The listing builds one solid part. Answer for the finished solid, in the listing's coordinates (mm). A direction names the side the tool comes from. Round coordinates to 2 decimals unless told otherwise and drop trailing zeros. Write each loop counter-clockwise with the first axis right and the second up, starting at its lowest first coordinate (ties: lowest second). Pieces come first, ordered by that corner, then holes. Notation, with made-up numbers: (-12, -24) - (36, -24) arc R20 ccw to (36, -5) - close; hole circle Ø2 at (46, -18). An arc over 180 degrees is marked (long way). Use a Markdown table: item, result. Add a question column.
1) A cutting plane is placed at D-D (y = -11.5). Give the vertices of the cut face in (x, z) (3 decimals).
2) Each of these flat-tipped pins is pushed along its axis until it touches: P1, Ø3, axis at x = 8, z = 4.62, coming from the -Y side; P2, Ø10, axis at y = 10.5, z = -8, coming from the -X side; P3, Ø6, axis at x = 8, z = -2, coming from the +Y side; P4, Ø6, axis at x = -5, y = 13.5, coming from the +Z side. Where does it stop, or does it pass through?
3) Determine the mould class of faces 1 (the flat face through (5, -11.04, 5)), 2 (the cylindrical face through (-0.1, 15.1, 2.5)), 3 (the flat face through (0, 17.56, 3)) for opening direction Y: +Y half, -Y half, draft (parallel to the pull), parting line (faces both ways), or undercut.
4) A tool of negligible diameter and unlimited length cuts with its end or side. For faces 4 (the flat face through (0, -17.56, -3)), 5 (the cylindrical face through (-1.951, 16.292, -6.195)), 6 (the cylindrical face through (3.955, -0.155, 5.158)), from which of +Z, -Z, +X, -X, +Y, -Y can it reach the whole face along a straight path? Write none if from no direction.
5) Find the intervals of material crossed by probe 1 along Y at (x, z) = (-4.75, -7.75); probe 2 along Z at (x, y) = (0.25, 4.5); probe 3 along X at (y, z) = (-12, 0.25), in increasing order. Write a range as from..to.
6) A cutting plane is placed at C-C (x = -8). Give the vertices of the cut face in (y, z).
```python
from build123d import *

# Parameters (mm, degrees)
FORO_FILETTATO_M3X0_5_1_D = 2.5


with BuildPart() as part:
    # Schizzo1 → Rivoluzione1 (revolve)
    with BuildSketch(Plane.XY, mode=Mode.PRIVATE) as rivoluzione1_sk:
        Polygon((2.5, -12.56), (4.5, -12.56), (4.5, 12.56), (2.5, 12.56), (2.5, 17.56), (6.495, 17.56), (6.495, 15.06), (12.485, 15.06), (12.485, 11.04), (6.5, 11.04), (6.5, -11.04), (12.485, -11.04), (12.485, -15.06), (6.495, -15.06), (6.495, -17.56), (2.5, -17.56), align=None)
    revolve(rivoluzione1_sk.sketch.rotate(Axis((0, 0, 0), (0, 1, 0)), 90), axis=Axis((0, 0, 0), (0, 1, 0)))

    # Foro filettato M3x0.5-1 (through all)
    with Locations(Plane(origin=(0, 15.06, 0), x_dir=(1, 0, 0), z_dir=(0, 1, 0))):
        with Locations((0, 9.237604307), (8, -4.618802154), (-8, -4.618802154)):
            Hole(FORO_FILETTATO_M3X0_5_1_D / 2)


solid = part.part
```
Entries:
| question | item | result |
|---|---|---|
| 1 | outline | circle Ø24.97 at (0, 0); hole circle Ø2.5 at (-8, 4.619); hole circle Ø9 at (0, 0); hole circle Ø2.5 at (0, -9.238); hole circle Ø2.5 at (8, 4.619) |
| 2 | P1 | stops at y = -15.06 |
| 2 | P2 | stops at x = -12.11 |
| 2 | P3 | stops at y = 17.56 |
| 2 | P4 | stops at z = 12.32 |
| 3 | face 1 | undercut |
| 3 | face 2 | draft |
| 3 | face 3 | +Y half |
| 4 | face 4 | +Z, -Z, +X, -X, -Y |
| 4 | face 5 | +Y |
| 4 | face 6 | none |
| 5 | probe 1 | y = -15.06..-11.04, 11.04..15.06 |
| 5 | probe 2 | z = -6.5..-4.49, 4.49..6.5 |
| 5 | probe 3 | x = -12.48..-4.49, 4.49..12.48 |
| 6 | outline | (-15.06, -9.59) - (-11.04, -9.59) - (-11.04, 3.37) - (-15.06, 3.37) - close; (-15.06, 5.87) - (-11.04, 5.87) - (-11.04, 9.59) - (-15.06, 9.59) - close; (11.04, -9.59) - (15.06, -9.59) - (15.06, 3.37) - (11.04, 3.37) - close; (11.04, 5.87) - (15.06, 5.87) - (15.06, 9.59) - (11.04, 9.59) - close |
